```python
from build123d import *

# Parameters (mm, degrees)
BOSS_EXTRUDE1_DEPTH = 14
FILLET1_R           = 3
SKETCH2_R           = 2.149999998
CUT_EXTRUDE1_DEPTH  = 20
BOSS_EXTRUDE2_START = 31.5
BOSS_EXTRUDE2_DEPTH = 31.5
FILLET2_R           = 3
SKETCH4_W           = 4.998300131
SKETCH4_H           = 5
BOSS_EXTRUDE3_DEPTH = 7
SKETCH5_W           = 10
SKETCH5_H           = 5
BOSS_EXTRUDE4_DEPTH = 4
FILLET3_R           = 1


with BuildPart() as part:
    # Sketch1 → Boss-Extrude1 (new body)
    with BuildSketch(Plane.XY):
        with BuildLine():
            Line((-1.241250307, 13.85672555), (-14.250633986, 13.85672555))
            Line((-14.250633986, 13.85672555), (-14.250633986, 17.85672555))
            Line((-14.250633986, 17.85672555), (-5.250633986, 17.85672555))
            ThreePointArc((-5.250633986, 17.85672555), (-3.129313642, 18.735405207), (-2.250633986, 20.85672555))
            Line((-2.250633986, 20.85672555), (-2.250633986, 59.910721228))
            Line((-2.250633986, 59.910721228), (-0.250633986, 59.910721228))
            Line((-0.250633986, 59.910721228), (45.249366014, 59.910721228))
            Line((45.249366014, 59.910721228), (55.360948415, 42.396946765))
            ThreePointArc((55.360948415, 42.396946765), (55.660649682, 41.673403901), (55.762872203, 40.896946765))
            Line((55.762872203, 40.896946765), (55.762872203, 18.148173952))
            ThreePointArc((55.762872203, 18.148173952), (55.061005533, 16.219811123), (53.283816736, 15.193750693))
            Line((53.283816736, 15.193750693), (40.181909711, 12.883530985))
            ThreePointArc((40.181909711, 12.883530985), (39.506607037, 12.680287949), (38.897409174, 12.325014256))
            Line((38.897409174, 12.325014256), (13.646499049, -6.702911338))
            ThreePointArc((13.646499049, -6.702911338), (11.449475402, -7.281339392), (9.477021718, -6.153989234))
            Line((9.477021718, -6.153989234), (-1.349799491, 7.703709976))
            ThreePointArc((-1.349799491, 7.703709976), (-2.398718311, 8.553107689), (-3.713831752, 8.85672555))
            Line((-3.713831752, 8.85672555), (-14.250633986, 8.85672555))
            Line((-14.250633986, 8.85672555), (-14.250633986, 12.85672555))
            Line((-14.250633986, 12.85672555), (-3.093333978, 12.85672555))
            Line((-3.093333978, 12.85672555), (-0.493883182, 12.85672555))
            ThreePointArc((-0.493883182, 12.85672555), (0.821230258, 12.553107689), (1.870149079, 11.703709976))
            Line((1.870149079, 11.703709976), (12.207057793, -1.526929835))
            Line((12.207057793, -1.526929835), (37.422217436, 17.474055838))
            Line((37.422217436, 17.474055838), (50.762872203, 19.826373214))
            Line((50.762872203, 19.826373214), (50.762872203, 39.578259723))
            Line((50.762872203, 39.578259723), (31.01448812, 44.86982329))
            Line((31.01448812, 44.86982329), (15.607892966, 29.463228136))
            Line((15.607892966, 29.463228136), (0.880070037, 14.735405207))
            ThreePointArc((0.880070037, 14.735405207), (-0.09320001, 14.085086953), (-1.241250307, 13.85672555))
        make_face()
        with BuildLine():
            Line((45.951332722, 48.694879226), (42.79562737, 54.160721228))
            ThreePointArc((42.79562737, 54.160721228), (42.246589264, 54.709759334), (41.496589264, 54.910721228))
            Line((41.496589264, 54.910721228), (24.253494556, 54.910721228))
            ThreePointArc((24.253494556, 54.910721228), (22.766327264, 53.606510517), (23.865265988, 51.961832489))
            Line((23.865265988, 51.961832489), (44.264066048, 46.495990486))
            ThreePointArc((44.264066048, 46.495990486), (45.842324626, 47.031737082), (45.951332722, 48.694879226))
        make_face(mode=Mode.SUBTRACT)
        with BuildLine():
            Line((23.600595455, 44.526998437), (5.310026186, 26.236429168))
            ThreePointArc((5.310026186, 26.236429168), (3.675340866, 25.911270041), (2.749366014, 27.29708934))
            Line((2.749366014, 27.29708934), (2.749366014, 50.488601873))
            ThreePointArc((2.749366014, 50.488601873), (3.336223871, 51.678631883), (4.637594582, 51.937490612))
            Line((4.637594582, 51.937490612), (22.92816385, 47.036547348))
            ThreePointArc((22.92816385, 47.036547348), (23.988824022, 45.975887176), (23.600595455, 44.526998437))
        make_face(mode=Mode.SUBTRACT)
    extrude(amount=-BOSS_EXTRUDE1_DEPTH)

    # Fillet1
    fillet1_edges = [part.edges().sort_by_distance(p)[0] for p in [
        (-2.250633986, 59.910721228, -7),
        (45.249366014, 59.910721228, -7),
    ]]
    fillet(fillet1_edges, radius=FILLET1_R)

    # Sketch2 → Cut-Extrude1 (cut)
    with BuildSketch(Plane.XZ.offset(-8.85672555)):
        with Locations((-9.950633986, -6.999923237)):
            Circle(SKETCH2_R)
    extrude(amount=-CUT_EXTRUDE1_DEPTH, mode=Mode.SUBTRACT)

    # Sketch3 → Boss-Extrude2 (add)
    with BuildSketch(Plane(origin=(0, 0, -14), x_dir=(-1, 0, 0), z_dir=(0, 0, -1)).offset(BOSS_EXTRUDE2_START)):
        with BuildLine():
            Line((-43.517315207, 59.910721228), (-0.749366014, 59.910721228))
            ThreePointArc((-0.749366014, 59.910721228), (1.371954329, 59.032041572), (2.250633986, 56.910721228))
            Line((2.250633986, 56.910721228), (2.250633986, 54.910721228))
            Line((2.250633986, 54.910721228), (-48.13611736, 54.910721228))
            Line((-48.13611736, 54.910721228), (-46.115391418, 58.410721228))
            ThreePointArc((-46.115391418, 58.410721228), (-45.017315207, 59.50879744), (-43.517315207, 59.910721228))
        make_face()
    extrude(amount=-BOSS_EXTRUDE2_DEPTH)

    # Fillet2
    # the kernel refuses this fillet: 3 mm, written as the material it takes off along each edge
    with BuildSketch(Plane(origin=(-2.250633986, 54.910721228, -52.571067812), x_dir=(0, 1, 0), z_dir=(0, 0, 1))) as fillet2_piece_1:
        with BuildLine():
            CenterArc((3, -2.828427125), FILLET2_R, 109.471220634, 70.528779366)
            Line((0, -2.828427125), (-0.06, -2.828427125))
            Line((-0.06, -2.828427125), (-0.06, 0))
            Line((-0.06, 0), (0, 0.06))
            ThreePointArc((0, 0.06), (1, 0.06), (1.98, 0.056568542))
            Line((1.98, 0.056568542), (2, 0))
        make_face()
    extrude(amount=38.571067812, mode=Mode.SUBTRACT)
    with BuildSketch(Plane(origin=(48.13611736, 54.910721228, -57.946914584), x_dir=(-1, 0, 0), z_dir=(0, 0, 1))) as fillet2_piece_2:
        with BuildLine():
            CenterArc((4.978765834, -3), FILLET2_R, 90, 99.594068227)
            Line((2.020725942, -3.5), (1.961565144, -3.51))
            ThreePointArc((1.961565144, -3.51), (0.958401447, -1.78), (-0.051961524, -0.03))
            Line((-0.051961524, -0.03), (0, 0.06))
            Line((0, 0.06), (4.978765834, 0.06))
            Line((4.978765834, 0.06), (4.978765834, 0))
        make_face()
    extrude(amount=43.946914584, mode=Mode.SUBTRACT)

    # Sketch4 → Boss-Extrude3 (add)
    with BuildSketch(Plane(origin=(0, 0, -14), x_dir=(-1, 0, 0), z_dir=(0, 0, -1))):
        with Locations((-0.24851608, 43.455333299)):
            Rectangle(SKETCH4_W, SKETCH4_H)
        Polygon((-9.274118244, 30.200521226), (-5.738584338, 26.66498732), (-9.274118244, 23.129453414), (-12.80965215, 26.66498732), align=None)
    extrude(amount=BOSS_EXTRUDE3_DEPTH)

    # Sketch5 → Boss-Extrude4 (add)
    with BuildSketch(Plane(origin=(0, 0, -21), x_dir=(-1, 0, 0), z_dir=(0, 0, -1))):
        Polygon((-12.80965215, 26.66498732), (-9.274118244, 23.129453414), (-2.203050432, 30.200521226), (-5.738584338, 33.736055132), align=None)
        with Locations((-2.749366014, 43.455333299)):
            Rectangle(SKETCH5_W, SKETCH5_H)
    extrude(amount=BOSS_EXTRUDE4_DEPTH)

    # Fillet3
    fillet3_edges = [part.edges().sort_by_distance(p)[0] for p in [
        (0.248516079, 40.955333299, -14),
        (0.248516079, 45.955333299, -14),
        (2.747666145, 43.455333299, -21),
        (11.041885197, 28.432754273, -14),
        (7.506351291, 24.897220367, -14),
        (7.506351291, 28.432754273, -21),
        (-2.250633986, 43.455333299, -25),
        (11.041885197, 24.897220367, -25),
    ]]
    fillet(fillet3_edges, radius=FILLET3_R)


solid = part.part
```
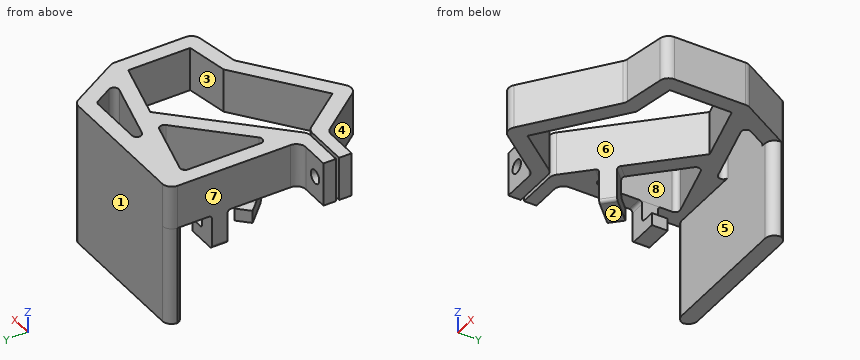
Check sheet for the modelled part. Datum: model origin and axes. Units: mm. Face numbers are marked on the shaded views. A direction names the side the tool comes from. Round coordinates to 2 decimals unless told otherwise and drop trailing zeros. Order: outer loops, then holes, each group sorted by start corner. A loop starts at its lowest first (then second) coordinate and runs counter-clockwise, first axis right, second up. Notation, with made-up numbers: M -33,63 L -14,63 A13 cw -14,83 Z; hole C 41.5,35 d7. An arc over 180 degrees is marked long. Answer in a Markdown table with one row per item.
(1) Draft check along Y on the marked faces 1, 2, 3 and 4. Enter one of: +Y half, -Y half, draft (parallel to the pull), parting line (faces both ways), or undercut.
Findings:
| item | result |
|---|---|
| face 1 | +Y half |
| face 2 | draft |
| face 3 | undercut |
| face 4 | -Y half |
(2) Section check C-C on z = -40.5. Record the boundary of the cut face in (x, y), plus the area to 3 significant figures.
Findings:
| item | result |
|---|---|
| outline | M -2.25,56.91 A3 ccw 0.58,54.91 L 43.16,54.91 A3 ccw 46.12,58.41 A3 ccw 43.52,59.91 L 0.75,59.91 A3 ccw Z |
| area | 235 mm^2 |
(3) Section check A-A on x = 30. Record the boundary of the cut face in (y, z).
Findings:
| item | result |
|---|---|
| outline | M 5.62,-14 L 11.88,-14 L 11.88,0 L 5.62,0 Z; M 43.86,-14 L 50.32,-14 L 50.32,0 L 43.86,0 Z; M 54.91,-45.5 L 59.91,-45.5 L 59.91,0 L 54.91,0 Z |
(4) Material ranges on line 1 along Y through (x, z) = (30.5, -8); line 2 along Y through (x, z) = (8, -5.5); line 3 along Y through (x, z) = (6, -38.5), recorded low to high. Write a range as from..to.
Findings:
| item | result |
|---|---|
| line 1 | y = 6..12.26, 44.36..50.18, 54.91..59.91 |
| line 2 | y = -4.26..3.86, 21.86..28.93, 51.04..59.91 |
| line 3 | y = 54.91..59.91 |
(5) Section check D-D on z = -13. Give the number of separate pieces and of enclosed holes in the cut face, plus the area to 3 significant figures.
Findings:
| item | result |
|---|---|
| separate pieces | 1 |
| enclosed holes | 2 |
| area | 1,510 mm^2 |
(6) Gauge pin test, flat ends, axial feed: pin 1 (5 mm diameter, centred on x = 5.5, y = 26.5, fed in from -Z); pin 2 (6.5 mm diameter, centred on y = 44, z = -17.5, fed in from +X); pin 3 (3 mm diameter, centred on y = 42.5, z = -22.5, fed in from +X). Record the tip position at first contact, or that the pin passes through.
Findings:
| item | result |
|---|---|
| pin 1 | stops at z = -25 |
| pin 2 | stops at x = 3.09 |
| pin 3 | stops at x = 7.75 |
(7) Set-up check for the marked faces 5, 6, 7 and 8: record each of +Z, -Z, +X, -X, +Y, -Y from which the full face is reachable in a straight line by a thin tool's end or side.
Findings:
| item | result |
|---|---|
| face 5 | -Z |
| face 6 | +Z, -Z |
| face 7 | +Z, -Z, -X, +Y |
| face 8 | +Z |
(8) Section check B-B on y = 35. Record the boundary of the cut face in (x, z).
Findings:
| item | result |
|---|---|
| outline | M -2.25,-14 L 2.75,-14 L 2.75,0 L -2.25,0 Z; M 14.07,-14 L 21.14,-14 L 21.14,0 L 14.07,0 Z; M 50.76,-14 L 55.76,-14 L 55.76,0 L 50.76,0 Z |
